```python
from build123d import *

# Parameters (mm, degrees)
F0_R     = 5
F1_DEPTH = 25
F3_DEPTH = 100.001
F4_SIZE  = 2


with BuildPart() as f1:
    # F0 (on Top) → F1 (new body)
    with BuildSketch(Plane.XY):
        with BuildLine():
            Line((45, 16.932883), (-45, 16.932883))
            ThreePointArc((-45, 16.932883), (-48.535534, 15.468417), (-50, 11.932883))
            Line((-50, 11.932883), (-50, 5))
            ThreePointArc((-50, 5), (-48.535534, 1.464466), (-45, 0))
            Line((-45, 0), (45, 0))
            ThreePointArc((45, 0), (48.535534, 1.464466), (50, 5))
            Line((50, 5), (50, 11.932883))
            ThreePointArc((50, 11.932883), (48.535534, 15.468417), (45, 16.932883))
        make_face()
        with Locations((-32.991346, 7.536008)):
            Circle(F0_R, mode=Mode.SUBTRACT)
    extrude(amount=F1_DEPTH)

    # F2 (on face) → F3 (cut, through all)
    with BuildSketch(Plane(origin=(-50, 0, 0), x_dir=(0, -1, 0), z_dir=(-1, 0, 0))):
        with BuildLine():
            ThreePointArc((-7.88945, 10.419369), (-6.747756, 11.19307), (-6.307288, 12.5))
            ThreePointArc((-6.307288, 12.5), (-7.159511, 14.218685), (-9.043432, 14.580631))
            Line((-9.043432, 14.580631), (-7.88945, 10.419369))
        make_face()
        with BuildLine():
            Line((-7.88945, 10.419369), (-9.043432, 14.580631))
            ThreePointArc((-9.043432, 14.580631), (-10.547073, 11.923009), (-7.88945, 10.419369))
        make_face()
    extrude(amount=-F3_DEPTH, mode=Mode.SUBTRACT)

    # F4
    f4_edges = [f1.edges().sort_by_distance(p)[0] for p in [
        (0, 16.932883, 25),
    ]]
    chamfer(f4_edges, length=F4_SIZE)


solid = f1.part
```
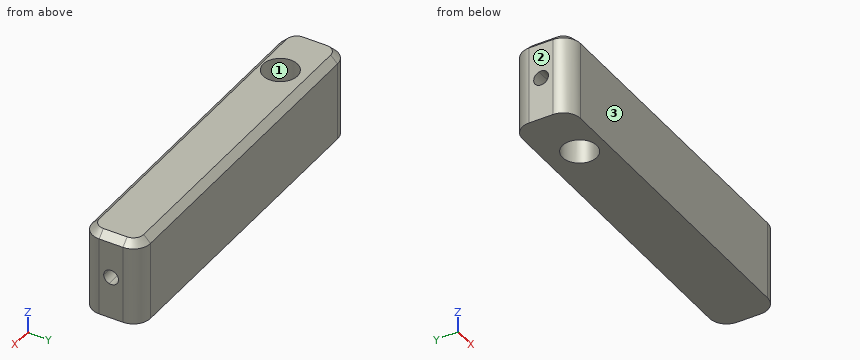
CAD build for the part. Positions are in the model's coordinates, mm. Face numbers are marked on the shaded views. Give positions to 0.01 mm unless a question says otherwise; leave off trailing zeros. Loops run counter-clockwise (first coordinate to the right, second up) from the corner with the lowest first, then second, coordinate; pieces in that order, holes last. Notation, with made-up numbers: M 59,28 L 103,28 A8 cw 103,32 Z; hole C 40,51.25 d4. An arc over 180 degrees is marked long. Use one line per item in the form item = value.
Item 1: Drill centre lines: probe 1 along X at (y, z) = (7.5, 22.75); probe 2 along X at (y, z) = (6, 20.75); probe 3 along Z at (x, y) = (-7, 8.75). Where is each one in solid material? Low to high. Write a range as from..to.
Determined:
probe_1 = -50..-37.99, -27.99..50
probe_2 = -50..-37.75, -28.23..50
probe_3 = 0..10.36, 14.64..25
Item 2: Slice it at A-A (x = 35). List the corners of the cut face in (y, z), plus the area to 3 significant figures.
Determined:
outline = M 0,0 L 16.93,0 L 16.93,23 L 14.93,25 L 2,25 L 0,23 Z; hole M 6.31,12.5 A2.16 ccw 7.89,10.42 A2.16 ccw 9.04,14.58 A2.16 ccw Z
area = 405 mm2
Item 3: Two-plate mould, pull along X, no slides. Class the marked faces 1, 2 and 3: pulls with the +X half, pulls with the -X half, needs draft (parallel to the pull), parting line crosses it, or undercut.
Determined:
face_1 = undercut
face_2 = pulls with the -X half
face_3 = needs draft
Item 4: Slice it at B-B (z = 19). List the corners of the cut face in (x, y), plus the area to 3 significant figures.
Determined:
outline = M -50,5 A5 ccw -45,0 L 45,0 A5 ccw 50,5 L 50,11.93 A5 ccw 45,16.93 L -45,16.93 A5 ccw -50,11.93 Z; hole C -32.99,7.54 d10
area = 1,590 mm2
